from build123d import *

# Parameters (mm, degrees)
F0_W     = 152.4
F0_H     = 63.5
F1_DEPTH = 25.4
F2_SIZE2 = 14.664687
F2_SIZE  = 25.39999
F3_SIZE2 = 14.664687
F3_SIZE  = 25.39999


# Not quite as in the source:
# - a fillet or chamfer is up to 0.001 mm smaller than in the source, because OpenCascade refuses the exact size


with BuildPart() as f1:
    # F0 (on Top) → F1 (new body)
    with BuildSketch(Plane.XY):
        with Locations((8.8605511625, -31.75)):
            Rectangle(F0_W, F0_H)
    extrude(amount=F1_DEPTH)

    # F2 (size 25.4 and 14.6646968374 in the source; OpenCascade refuses exactly that, so slightly less here)
    f2_edges = [f1.edges().sort_by_distance(p)[0] for p in [
        (85.060551, -31.75, 25.4),
    ]]
    f2_side = f1.faces().sort_by_distance((85.060551, -31.75, 12.7))[0]
    chamfer(f2_edges, length=F2_SIZE, length2=F2_SIZE2, reference=f2_side)

    # F3 (size 25.4 and 14.6646968374 in the source; OpenCascade refuses exactly that, so slightly less here)
    f3_edges = [f1.edges().sort_by_distance(p)[0] for p in [
        (-67.339449, -31.75, 0),
    ]]
    f3_side = f1.faces().sort_by_distance((-67.339449, -31.75, 12.7))[0]
    chamfer(f3_edges, length=F3_SIZE, length2=F3_SIZE2, reference=f3_side)


solid = f1.part
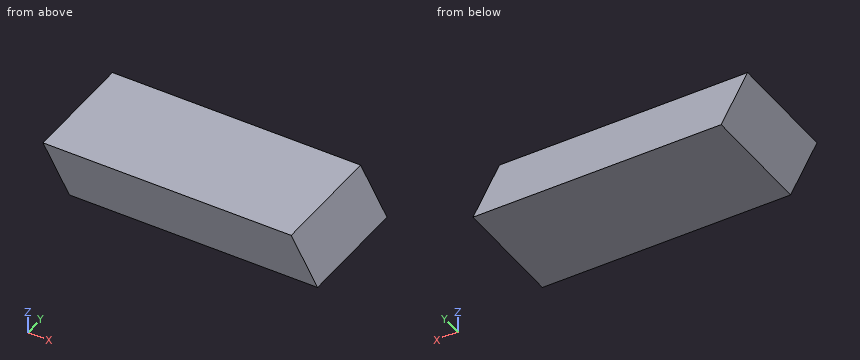
The model under review builds one solid part; all positions refer to its coordinate system, in mm. Coordinates: 2 decimals unless noted, no trailing zeros. Loops run counter-clockwise (first coordinate to the right, second up) from the corner with the lowest first, then second, coordinate; pieces in that order, holes last. Notation, with made-up numbers: M 31.25,-12 L 59.25,-12 A9 ccw 59.25,-1 Z; hole C 27,63 d3. An arc over 180 degrees is marked long. Put each result on its own line as item: value. Start each with the question number.
Q1. Wall thickness on line 1 (X direction, y = -38.5, z = 3.75); line 2 (X direction, y = -17.5, z = 15.5); line 3 (Z direction, x = -60.5, y = -28.5): over which ranges is each line inside the solid? List them lowest first.
Q2. Clearance check with flat-ended pins moving along their axes: pin 1 (5 mm diameter, centred on y = -53.5, z = 19, fed in from -X); pin 2 (10 mm diameter, centred on y = -18.5, z = 13.5, fed in from -X). State where each tip first meets the part, or that it passes through.
Q3. Add section B-B (z = 23). Write out the cut boundary in (x, y), and give its area (3 significant figures).
Answers:
1. line 1: x = -54.84 to 82.9
1. line 2: x = -61.62 to 76.11
1. line 3: z = 13.55 to 25.4
2. pin 1: stops at x = -65.09
2. pin 2: stops at x = -63.36
3. outline: M -65.95,-63.5 L 71.78,-63.5 L 71.78,0 L -65.95,0 Z
3. area: 8,750 mm^2
